```python
from build123d import *

# Parameters (mm, degrees)
KEYED_BACK_DEPTH   = 0.5
CUP_BLANK_SKETCH_R = 3.8
CUP_BLANK_DEPTH    = 1.5


with BuildPart() as part:
    # Keyed Back Sketch → Keyed Back (new body)
    with BuildSketch(Plane(origin=(0, -69, 0), x_dir=(-1, 0, 0), z_dir=(0, -1, 0))):
        with BuildLine():
            Line((23.291651246, 2.332380758), (23.291651246, -2.332380758))
            ThreePointArc((23.291651246, -2.332380758), (30.091651246, 0), (23.291651246, 2.332380758))
        make_face()
    extrude(amount=KEYED_BACK_DEPTH)

    # Cup Blank Sketch → Cup Blank (add)
    with BuildSketch(Plane(origin=(0, -69.5, 0), x_dir=(-1, 0, 0), z_dir=(0, -1, 0))):
        with Locations(Location((26.291651246, 0, 0), (0, 0, 217.863646362))):
            Circle(CUP_BLANK_SKETCH_R)
    extrude(amount=CUP_BLANK_DEPTH)

    # Spherical Bearing Seat profile → Spherical Bearing Seat (revolve, cut)
    with BuildSketch(Plane(origin=(0, -73, 0), x_dir=(-1, 0, 0), z_dir=(0, -1, 0))):
        with BuildLine():
            Line((26.291651246, -3.1), (26.291651246, 3.1))
            ThreePointArc((26.291651246, 3.1), (23.191651246, 0), (26.291651246, -3.1))
        make_face()
    revolve(axis=Axis((-26.291651246, -73, -10), (0, 0, 1)), mode=Mode.SUBTRACT)


with BuildPart() as body_2:
    # Mirror1: mirrored copy
    add(part.part.mirror(Plane(origin=(0, 0, 0), x_dir=(0, 0, 1), z_dir=(0, -1, 0))))


solid = body_2.part
```
Verification items for the finished model (mm, model axes). A direction names the side the tool comes from. Round coordinates to 2 decimals unless told otherwise and drop trailing zeros. Order: outer loops, then holes, each group sorted by start corner. A loop starts at its lowest first (then second) coordinate and runs counter-clockwise, first axis right, second up. Notation, with made-up numbers: (-23.75, -19.5) -> (-6.75, -19.5) arc R20 cw to (-6.75, -1.5) -> close; hole circle Ø2 at (48.5, 19.5). An arc over 180 degrees is marked (long way). Put each result on its own line as item: value. Start each with the question number.
(1) Section check A-A (z = 1). Enter the section's corners in (x, y), then the cut area to 3 significant figures.
(2) Tool access check on faces 1 (the face through (-24, 71, 2)), 2 (the face through (-23, 69.5, 0)). Record the directions out of +Z, -Z, +X, -X, +Y, -Y that give a thin tool (end or side, any length) a straight path to the whole face; none if there is none.
(3) Section check B-B (y = 69.65). Enter the section's corners in (x, z), then the cut area to 3 significant figures.
(4) Depth check by flat-ended pin: pin 1 Ø1 at (x, y) = (-25, 69) entering from +Z. Enter the tip coordinate at first touch or a pass-through.
(5) Section check C-C (x = -28). Enter the section's corners in (y, z).
(6) Material ranges on line 1 along Y through (x, z) = (-22.75, -1); line 2 along Z through (x, y) = (-27, 70.6); line 3 along Z through (x, y) = (-28.75, 69.5), recorded low to high.
(7) Section check D-D (z = -2.5). Enter the section's corners in (x, y).
Completed:
1. outline: (-29.96, 69) -> (-23.29, 69) -> (-23.29, 69.5) -> (-22.63, 69.5) -> (-22.63, 71) -> (-24.14, 71) arc R2.93 cw to (-28.44, 71) -> (-29.96, 71) -> close
1. area: 11.6 mm2
2. face 1: +Z, -Z, +X, -X, +Y
2. face 2: +Z, -Z, +X, -Y
3. outline: circle Ø7.6 at (-26.29, 0)
3. area: 45.4 mm2
4. pin 1: stops at z = 3.72
5. outline: (69, -3.39) -> (71, -3.39) -> (71, -1.64) arc R2.59 cw to (71, 1.64) -> (71, 3.39) -> (69, 3.39) -> close
6. line 1: y = 69.5 to 71
6. line 2: z = -3.73 to -1.83, 1.83 to 3.73
6. line 3: z = -2.9 to 2.9
7. outline: (-29.15, 69) -> (-23.43, 69) -> (-23.43, 71) -> (-29.15, 71) -> close
